from build123d import *

# Parameters (mm, degrees)
BLOCK_DEPTH                    = 110
SHELL1_T                       = -3
SKETCH2_R                      = 5
CORNER_COLUMNS_DEPTH           = 110
SKETCH3_R                      = 2
FRONT_PANEL_INSERT_HOLES_DEPTH = 7
SKETCH4_R                      = 4.5
PLATE_BOSSES_DEPTH             = 6
SKETCH5_R                      = 2
PLATE_INSERT_HOLES_DEPTH       = 7
SKETCH6_R                      = 8.15
SKETCH6_R_2                    = 6.4
CABLE_GLAND_HOLES_DEPTH        = 4
SKETCH7_W                      = 12
SKETCH7_H                      = 6
CABLE_TIE_BARS_DEPTH           = 12
SKETCH8_W                      = 4
SKETCH8_H                      = 2.5
CABLE_TIE_SLOTS_DEPTH          = 6.02
SKETCH9_W                      = 14
SKETCH9_H                      = 14
USB_ACCESS_DEPTH               = 4
VENTS_LEFT_DEPTH               = 4
VENTS_START                    = -4
VENTS_RIGHT_DEPTH              = 4
SKETCH12_R                     = 4.75
KEYHOLE_HEADS_DEPTH            = 4
KEYHOLE_SLOTS_DEPTH            = 4
SKETCH14_W                     = 24
SKETCH14_H                     = 16
WALL_EARS_DEPTH                = 5
SKETCH15_R                     = 2.15
WALL_EAR_SCREW_HOLES_DEPTH     = 266.331867668


with BuildPart() as part:
    # Sketch1 → Block (new body)
    with BuildSketch(Plane.XY):
        with BuildLine():
            Line((-77, 0), (77, 0))
            ThreePointArc((77, 0), (82.656854249, 2.343145751), (85, 8))
            Line((85, 8), (85, 202))
            ThreePointArc((85, 202), (82.656854249, 207.656854249), (77, 210))
            Line((77, 210), (-77, 210))
            ThreePointArc((-77, 210), (-82.656854249, 207.656854249), (-85, 202))
            Line((-85, 202), (-85, 8))
            ThreePointArc((-85, 8), (-82.656854249, 2.343145751), (-77, 0))
        make_face()
    extrude(amount=BLOCK_DEPTH)

    # Shell1
    shell1_openings = [part.faces().sort_by_distance(p)[0] for p in [
        (0, 105, 110),
    ]]
    offset(amount=SHELL1_T, openings=shell1_openings, kind=Kind.INTERSECTION)

    # Sketch2 → Corner columns (add)
    with BuildSketch(Plane.XY):
        with Locations((-78, 7)):
            Circle(SKETCH2_R)
        with Locations((78, 7)):
            Circle(SKETCH2_R)
        with Locations((-78, 203)):
            Circle(SKETCH2_R)
        with Locations((78, 203)):
            Circle(SKETCH2_R)
    extrude(amount=CORNER_COLUMNS_DEPTH)

    # Sketch3 → Front panel insert holes (cut)
    with BuildSketch(Plane.XY.offset(110)):
        with Locations((-78, 7)):
            Circle(SKETCH3_R)
        with Locations((78, 7)):
            Circle(SKETCH3_R)
        with Locations((-78, 203)):
            Circle(SKETCH3_R)
        with Locations((78, 203)):
            Circle(SKETCH3_R)
    extrude(amount=-FRONT_PANEL_INSERT_HOLES_DEPTH, mode=Mode.SUBTRACT)

    # Sketch4 → Plate bosses (add)
    with BuildSketch(Plane.XY.offset(3)):
        with Locations((-65, 46)):
            Circle(SKETCH4_R)
        with Locations((65, 46)):
            Circle(SKETCH4_R)
        with Locations((-65, 190)):
            Circle(SKETCH4_R)
        with Locations((65, 190)):
            Circle(SKETCH4_R)
    extrude(amount=PLATE_BOSSES_DEPTH)

    # Sketch5 → Plate insert holes (cut)
    with BuildSketch(Plane.XY.offset(9)):
        with Locations((-65, 46)):
            Circle(SKETCH5_R)
        with Locations((65, 46)):
            Circle(SKETCH5_R)
        with Locations((-65, 190)):
            Circle(SKETCH5_R)
        with Locations((65, 190)):
            Circle(SKETCH5_R)
    extrude(amount=-PLATE_INSERT_HOLES_DEPTH, mode=Mode.SUBTRACT)

    # Sketch6 → Cable gland holes (cut)
    with BuildSketch(Plane(origin=(0, 0, 0), x_dir=(1, 0, 0), z_dir=(0, 1, 0))):
        with Locations(Location((-50, -45, 0), (0, 0, 270))):
            Circle(SKETCH6_R)
        with Locations(Location((-15, -45, 0), (0, 0, 270))):
            Circle(SKETCH6_R_2)
        with Locations(Location((15, -45, 0), (0, 0, 270))):
            Circle(SKETCH6_R_2)
        with Locations(Location((50, -45, 0), (0, 0, 270))):
            Circle(SKETCH6_R_2)
    extrude(amount=CABLE_GLAND_HOLES_DEPTH, mode=Mode.SUBTRACT)

    # Sketch7 → Cable tie bars (add)
    with BuildSketch(Plane.XY.offset(3)):
        with Locations((-50, 30)):
            Rectangle(SKETCH7_W, SKETCH7_H)
        with Locations((-15, 30)):
            Rectangle(SKETCH7_W, SKETCH7_H)
        with Locations((15, 30)):
            Rectangle(SKETCH7_W, SKETCH7_H)
        with Locations((50, 30)):
            Rectangle(SKETCH7_W, SKETCH7_H)
    extrude(amount=CABLE_TIE_BARS_DEPTH)

    # Sketch8 → Cable tie slots (cut)
    with BuildSketch(Plane(origin=(0, 26.99, 0), x_dir=(1, 0, 0), z_dir=(0, 1, 0))):
        with Locations((-50, -10)):
            Rectangle(SKETCH8_W, SKETCH8_H)
        with Locations((-15, -10)):
            Rectangle(SKETCH8_W, SKETCH8_H)
        with Locations((15, -10)):
            Rectangle(SKETCH8_W, SKETCH8_H)
        with Locations((50, -10)):
            Rectangle(SKETCH8_W, SKETCH8_H)
    extrude(amount=CABLE_TIE_SLOTS_DEPTH, mode=Mode.SUBTRACT)

    # Sketch9 → USB access (cut)
    with BuildSketch(Plane(origin=(-85, 0, 0), x_dir=(0, 0, -1), z_dir=(1, 0, 0))):
        with Locations((-18, 95)):
            Rectangle(SKETCH9_W, SKETCH9_H)
    extrude(amount=USB_ACCESS_DEPTH, mode=Mode.SUBTRACT)

    # Sketch10 → Vents left (cut)
    with BuildSketch(Plane(origin=(-85, 0, 0), x_dir=(0, 0, -1), z_dir=(1, 0, 0))):
        with BuildLine():
            Line((-25, 170.5), (-65, 170.5))
            ThreePointArc((-65, 170.5), (-66.5, 172), (-65, 173.5))
            Line((-65, 173.5), (-25, 173.5))
            ThreePointArc((-25, 173.5), (-23.5, 172), (-25, 170.5))
        make_face()
        with BuildLine():
            Line((-25, 178.5), (-65, 178.5))
            ThreePointArc((-65, 178.5), (-66.5, 180), (-65, 181.5))
            Line((-65, 181.5), (-25, 181.5))
            ThreePointArc((-25, 181.5), (-23.5, 180), (-25, 178.5))
        make_face()
        with BuildLine():
            Line((-25, 186.5), (-65, 186.5))
            ThreePointArc((-65, 186.5), (-66.5, 188), (-65, 189.5))
            Line((-65, 189.5), (-25, 189.5))
            ThreePointArc((-25, 189.5), (-23.5, 188), (-25, 186.5))
        make_face()
    extrude(amount=VENTS_LEFT_DEPTH, mode=Mode.SUBTRACT)

    # Sketch11 → Vents right (cut)
    with BuildSketch(Plane(origin=(85, 0, 0), x_dir=(0, 0, -1), z_dir=(1, 0, 0)).offset(VENTS_START)):
        with BuildLine():
            Line((-25, 170.5), (-65, 170.5))
            ThreePointArc((-65, 170.5), (-66.5, 172), (-65, 173.5))
            Line((-65, 173.5), (-25, 173.5))
            ThreePointArc((-25, 173.5), (-23.5, 172), (-25, 170.5))
        make_face()
        with BuildLine():
            Line((-25, 178.5), (-65, 178.5))
            ThreePointArc((-65, 178.5), (-66.5, 180), (-65, 181.5))
            Line((-65, 181.5), (-25, 181.5))
            ThreePointArc((-25, 181.5), (-23.5, 180), (-25, 178.5))
        make_face()
        with BuildLine():
            Line((-25, 186.5), (-65, 186.5))
            ThreePointArc((-65, 186.5), (-66.5, 188), (-65, 189.5))
            Line((-65, 189.5), (-25, 189.5))
            ThreePointArc((-25, 189.5), (-23.5, 188), (-25, 186.5))
        make_face()
    extrude(amount=VENTS_RIGHT_DEPTH, mode=Mode.SUBTRACT)

    # Sketch12 → Keyhole heads (cut)
    with BuildSketch(Plane.XY):
        with Locations((-45, 165)):
            Circle(SKETCH12_R)
        with Locations((45, 165)):
            Circle(SKETCH12_R)
    extrude(amount=KEYHOLE_HEADS_DEPTH, mode=Mode.SUBTRACT)

    # Sketch13 → Keyhole slots (cut)
    with BuildSketch(Plane.XY):
        with BuildLine():
            Line((-47.15, 165), (-47.15, 176))
            ThreePointArc((-47.15, 176), (-45, 178.15), (-42.85, 176))
            Line((-42.85, 176), (-42.85, 165))
            ThreePointArc((-42.85, 165), (-45, 162.85), (-47.15, 165))
        make_face()
        with BuildLine():
            Line((42.85, 165), (42.85, 176))
            ThreePointArc((42.85, 176), (45, 178.15), (47.15, 176))
            Line((47.15, 176), (47.15, 165))
            ThreePointArc((47.15, 165), (45, 162.85), (42.85, 165))
        make_face()
    extrude(amount=KEYHOLE_SLOTS_DEPTH, mode=Mode.SUBTRACT)

    # Sketch14 → Wall ears (add)
    with BuildSketch(Plane.XY):
        with Locations((-55, -8)):
            Rectangle(SKETCH14_W, SKETCH14_H)
        with Locations((-55, 218)):
            Rectangle(SKETCH14_W, SKETCH14_H)
        with Locations((55, -8)):
            Rectangle(SKETCH14_W, SKETCH14_H)
        with Locations((55, 218)):
            Rectangle(SKETCH14_W, SKETCH14_H)
    extrude(amount=WALL_EARS_DEPTH)

    # Sketch15 → Wall ear screw holes (cut, through all)
    with BuildSketch(Plane.XY):
        with Locations(Location((-55, -8, 0), (0, 0, 180))):
            Circle(SKETCH15_R)
        with Locations(Location((-55, 218, 0), (0, 0, 180))):
            Circle(SKETCH15_R)
        with Locations(Location((55, -8, 0), (0, 0, 180))):
            Circle(SKETCH15_R)
        with Locations(Location((55, 218, 0), (0, 0, 180))):
            Circle(SKETCH15_R)
    extrude(amount=WALL_EAR_SCREW_HOLES_DEPTH, mode=Mode.SUBTRACT)


solid = part.part
Work out the finished part from the listing and answer in its coordinate system (mm). A direction names the side the tool comes from. Give positions to 0.01 mm unless a question says otherwise; leave off trailing zeros. Order: outer loops, then holes, each group sorted by start corner. A loop starts at its lowest first (then second) coordinate and runs counter-clockwise, first axis right, second up. Notation, with made-up numbers: (-13.5, -7.5) -> (28.5, -7.5) arc R21 cw to (28.5, 27.5) -> close; hole circle Ø4 at (63, 80.25). An arc over 180 degrees is marked (long way). Answer as a JSON object with one key per item and string values. Group by question number.
1. Section B-B on z = 29 is taken. Count the separate pieces of the cut face and the enclosed holes in it, plus the area to 3 significant figures.
2. Consider line 1 along Y through (x, z) = (-65, 4.5); line 2 along Y through (x, z) = (65, 7.5); line 3 along Y through (x, z) = (5.5, 37). Determine where each line is inside the solid, lowest interval first. Write a range as [from, to].
3. Section A-A on y = 165 is taken. Determine the outline of the cut face in (x, z).
4. Flat-ended cylindrical pins translate along their axes: pin 1 Ø5 at (x, y) = (-50.5, 217) entering from +Z; pin 2 Ø16.5 at (x, z) = (15, 45) entering from -Y; pin 3 Ø5 at (x, y) = (49.5, 54) entering from +Z; pin 4 Ø2.5 at (x, y) = (55, 218) entering from +Z. Find the tip coordinate at first contact, or state that the pin passes through.
5. A tool of negligible diameter and unlimited length cuts with its end or side. For faces 1 (the flat face through (-43, -8, 2)), 2 (the flat face through (-58, 218, 5)), 3 (the flat face through (67, 218, 2)), from which of +Z, -Z, +X, -X, +Y, -Y can it reach the whole face along a straight path? Write none if from no direction.
6. Section C-C on x = -25.5 is taken. Determine the outline of the cut face in (y, z), plus the area to 3 significant figures.
7. Section D-D on y = 22 is taken. Determine the outline of the cut face in (x, z), plus the area to 3 significant figures.
Result sheet:
{
 "1": {"separate pieces": "6", "enclosed holes": "0", "area": "2,420 mm^2"},
 "2": {"line 1": "y = [-16, 3], [41.5, 44], [48, 50.5], [185.5, 188], [192, 194.5], [207, 226]", "line 2": "y = [0, 3], [41.5, 44], [48, 50.5], [185.5, 188], [192, 194.5], [207, 210]", "line 3": "y = [0, 3], [207, 210]"},
 "3": {"outline": "(-85, 0) -> (-49.75, 0) -> (-49.75, 3) -> (-82, 3) -> (-82, 110) -> (-85, 110) -> close; (-40.25, 0) -> (40.25, 0) -> (40.25, 3) -> (-40.25, 3) -> close; (49.75, 0) -> (85, 0) -> (85, 110) -> (82, 110) -> (82, 3) -> (49.75, 3) -> close"},
 "4": {"pin 1": "stops at z = 5", "pin 2": "stops at y = 0", "pin 3": "stops at z = 3", "pin 4": "passes through"},
 "5": {"face 1": "+Z, -Z, -Y", "face 2": "+Z, +X, -X, +Y", "face 3": "+Z, -Z, +X, +Y"},
 "6": {"outline": "(0, 0) -> (210, 0) -> (210, 110) -> (207, 110) -> (207, 3) -> (3, 3) -> (3, 110) -> (0, 110) -> close", "area": "1,270 mm^2"},
 "7": {"outline": "(-85, 0) -> (85, 0) -> (85, 110) -> (82, 110) -> (82, 3) -> (-82, 3) -> (-82, 110) -> (-85, 110) -> close", "area": "1,150 mm^2"}
}
